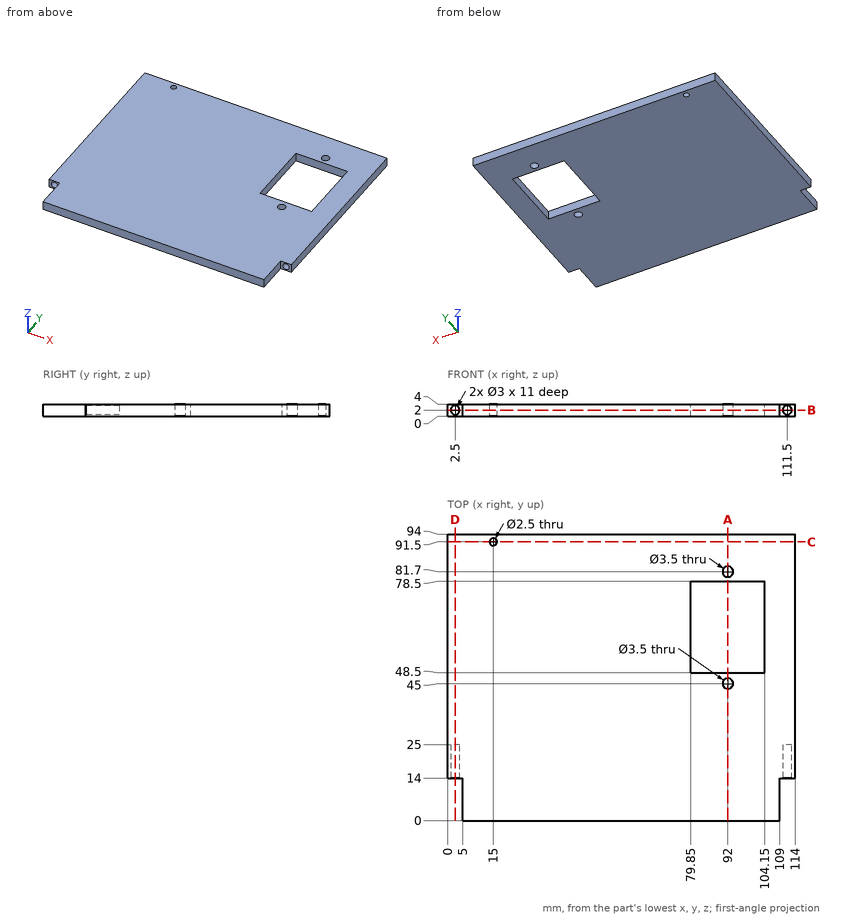
Could you check a few things on this drawing? It's one solid part, dimensions in mm from its lowest x, y, z. Give positions to 0.01 mm unless a question says otherwise; leave off trailing zeros. Loops run counter-clockwise (first coordinate to the right, second up) from the corner with the lowest first, then second, coordinate; pieces in that order, holes last. Notation, with made-up numbers: M -16.5,-36 L 38.5,-36 A20 ccw 38.5,-1 Z; hole C 25,31.25 d7. An arc over 180 degrees is marked long. Return JSON: item names as keys, results as strings.
Item 1: Imagine slicing it at C-C on y = 91.5. List the corners of the cut face in (x, z) for me, then the cut area to 3 significant figures.
A:
{"outline": "M 0,0 L 13.75,0 L 13.75,4 L 0,4 Z; M 16.25,0 L 114,0 L 114,4 L 16.25,4 Z", "area": "446 mm^2"}
Item 2: Imagine slicing it at D-D on x = 2.5. List the corners of the cut face in (y, z) for me, then the cut area to 3 significant figures.
A:
{"outline": "M 14,0 L 94,0 L 94,4 L 14,4 L 14,3.5 L 25,3.5 L 25,0.5 L 14,0.5 Z", "area": "287 mm^2"}
Item 3: Imagine slicing it at A-A on x = 92. List the corners of the cut face in (y, z) for me.
A:
{"outline": "M 0,0 L 43.25,0 L 43.25,4 L 0,4 Z; M 46.75,0 L 48.5,0 L 48.5,4 L 46.75,4 Z; M 78.5,0 L 79.95,0 L 79.95,4 L 78.5,4 Z; M 83.45,0 L 94,0 L 94,4 L 83.45,4 Z"}
Item 4: Please list where these lines run through material, in increasing order: line 1 (Y direction, x = 92, z = 2); line 2 (Y direction, x = 99, z = 2.25); line 3 (Y direction, x = 15, z = 1.3).
A:
{"line 1": "y = 0 to 43.25, 46.75 to 48.5, 78.5 to 79.95, 83.45 to 94", "line 2": "y = 0 to 48.5, 78.5 to 94", "line 3": "y = 0 to 90.25, 92.75 to 94"}
Item 5: I'm going to push flat-ended pins straight in: pin 1 Ø1.2 at (x, z) = (2, 2) entering from -Y; pin 2 Ø3 at (x, y) = (92, 45) entering from +Z; pin 3 Ø12 at (x, y) = (64.5, 83.5) entering from -Z; pin 4 Ø1.2 at (y, z) = (3.5, 1.5) entering from -X. Where does each tip first touch, or does it pass through?
A:
{"pin 1": "stops at y = 25", "pin 2": "passes through", "pin 3": "stops at z = 0", "pin 4": "stops at x = 5"}
Item 6: Imagine slicing it at B-B on z = 2. List the corners of the cut face in (x, y) for me, then the cut area to 3 significant figures.
A:
{"outline": "M 0,14 L 1,14 L 1,25 L 4,25 L 4,14 L 5,14 L 5,0 L 109,0 L 109,14 L 110,14 L 110,25 L 113,25 L 113,14 L 114,14 L 114,94 L 0,94 Z; hole C 15,91.5 d2.5; hole M 79.85,48.5 L 104.15,48.5 L 104.15,78.5 L 79.85,78.5 Z; hole C 92,45 d3.5; hole C 92,81.7 d3.5", "area": "9,760 mm^2"}
